The listing builds one solid part. Answer for the finished solid, in the listing's coordinates (mm). A direction names the side the tool comes from. Give positions to 0.01 mm unless a question says otherwise; leave off trailing zeros. Loops run counter-clockwise (first coordinate to the right, second up) from the corner with the lowest first, then second, coordinate; pieces in that order, holes last. Notation, with made-up numbers: M 73,-1 L 106,-1 A31 cw 106,29 Z; hole C 4.25,-22 d10. An arc over 180 degrees is marked long. One line per item, written item: value. Start each with the question number.
Q1. A cutting plane is placed at B-B, the plane x = 11. State how many separate pieces and enclosed holes the cut face has, and give its area (3 significant figures).
Q2. For faces 1 (the cylindrical face through (-6.852, 6.283, 29.088)), 2 (the flat face through (1, 1, 0)), determine the directions among +Z, -Z, +X, -X, +Y, -Y from which every point of the face is accessible in a straight line to the end or side of a thin tool.
Q3. A cutting plane is placed at A-A, the plane z = 61.5. Determine the outline of the cut face in (x, y).
Q4. Consider L1, parallel to Z at x = 16, y = -33; L2, parallel to Y at x = 0.5, z = 63.5; L3, parallel to Z at x = -3, y = -12. Determine where each line is inside the solid, lowest interval first.
Q5. Flat-ended cylindrical pins translate along their axes: pin 1 (12 mm diameter, centred on x = 14, z = 12, fed in from -Y); pin 2 (5 mm diameter, centred on x = -10, z = 19, fed in from +Y); pin 3 (2 mm diameter, centred on y = -8, z = 67, fed in from +X). Find the tip coordinate at first contact, or state that the pin passes through.
from build123d import *


with BuildPart() as f1:
    # F0 (on Front) → F1 (revolve)
    with BuildSketch(Plane.XZ):
        with BuildLine():
            Line((0, 74.917264), (0, 0))
            Line((0, 0), (39.240602, 0))
            ThreePointArc((39.240602, 0), (42.776984, 3.536382), (39.240602, 7.072763))
            ThreePointArc((39.240602, 7.072763), (22.703598, 9.45647), (9.296888, 19.427162))
            Line((9.296888, 19.427162), (9.296888, 38.482253))
            ThreePointArc((9.296888, 38.482253), (13.546492, 45.601735), (9.296888, 52.721217))
            Line((9.296888, 52.721217), (9.296888, 65.913208))
            ThreePointArc((9.296888, 65.913208), (13.798916, 70.415236), (9.296888, 74.917264))
            Line((9.296888, 74.917264), (0, 74.917264))
        make_face()
    revolve(axis=Axis((0, 0, 37.458632), (0, 0, 1)))


solid = f1.part
Answer block:
1. separate pieces: 3
1. enclosed holes: 0
1. area: 1,120 mm^2
2. face 1: none
2. face 2: -Z, +X, -X, +Y, -Y
3. outline: C 0,0 d18.59
4. L1: 0 to 6.9
4. L2: -9.28 to 9.28
4. L3: 0 to 16.13, 41.4 to 49.8, 67.12 to 73.71
5. pin 1: y = -39.65
5. pin 2: y = 7.71
5. pin 3: x = 10.64
